Design review of the part built by this model. Coordinates are the model's own, in mm. A direction names the side the tool comes from. Coordinates: 2 decimals unless noted, no trailing zeros. Order: outer loops, then holes, each group sorted by start corner. A loop starts at its lowest first (then second) coordinate and runs counter-clockwise, first axis right, second up. Notation, with made-up numbers: M 42.25,-30 L 51.25,-30 A8 cw 51.25,-18 Z; hole C -19.75,-28.75 d9. An arc over 180 degrees is marked long. Answer in a Markdown table with one row per item.
Autodesk Inventor part; units mm, degrees
ref_plane "Work Plane1" through (0, 21, 0) normal (0, 1, 0) x (1, 0, 0)
ref_plane "YZ Plane" through (0, 0, 0) normal (1, 0, 0) x (0, 1, 0)
ref_plane "XZ Plane" through (0, 0, 0) normal (0, 1, 0) x (-1, 0, 0)
sketch "Sketch1" plane through (0, 0, 0) normal (0, 1, 0) x (-1, 0, 0)
  line L0 (0, 0) -> (20, 0)
  line L1 (20, 0) -> (20, -20)
  line L2 (20, -20) -> (0, -20)
  line L3 (0, -20) -> (0, 0)
  dimension "d0" = 20
  dimension "d1" = 20
extrude "Extrusion1" add sketch "Sketch1" along normal blind 5
sketch "Sketch2" plane through (0, 5, 0) normal (0, 1, 0) x (1, 0, 0)
  line L0 (0, 0) -> (0, 20)
  line L1 (-20, 0) -> (0, 0)
  point P0 (-7.5, 5)
  dimension "d4" = 7.5
  dimension "d55" = 5
hole "Hole1" at (-7.5, 5, -5) direction (0, -1, 0) diameter 6.6 end through all
chamfer "Chamfer1" distance 0.5 angle 45 1 edges at (-7.5, 0, -8.3)
sketch "Sketch3" plane through (0, 5, 0) normal (0, 1, 0) x (1, 0, 0)
  circle A0 centre (-7.5, 5) radius 3.3 construction
  line L0 (0, 20) -> (-20, 20) construction
  line L1 (-20, 20) -> (-20, 0) construction
  line L2 (-20, 0) -> (0, 0) construction
  line L3 (0, 0) -> (0, 20) construction
  line L4 (-20, 20) -> (-20, 0) construction
  line L5 (0, 20) -> (-20, 20) construction
  line L6 (-20, 0) -> (-15, 0)
  line L7 (-15, 0) -> (-15, 20)
  line L8 (-15, 20) -> (-20, 20)
  line L9 (-20, 20) -> (-20, 0)
  line L10 (0, 20) -> (-20, 20)
  line L11 (-20, 20) -> (-20, 10)
  line L12 (-20, 10) -> (0, 10)
  line L13 (0, 10) -> (0, 20)
  point P0 (-15, 10)
  dimension "d56" = 15
  dimension "d57" = 10
extrude "Extrusion2" add sketch "Sketch3" along normal blind 15
sketch "Sketch6" plane through (0, 20, 0) normal (0, 1, 0) x (1, 0, 0)
  line L0 (0, 20) -> (-20, 20) construction
  line L1 (-20, 20) -> (-20, 0) construction
  line L2 (-20, 0) -> (-15, 0) construction
  line L3 (-15, 0) -> (-15, 10) construction
  line L4 (-15, 10) -> (0, 10) construction
  line L5 (0, 10) -> (0, 20) construction
  line L6 (-2.5, 10) -> (-13, 10)
  line L7 (-13, 10) -> (-13, 20)
  line L8 (-13, 20) -> (-2.5, 20)
  line L9 (-2.5, 20) -> (-2.5, 10)
  dimension "d32" = 2.5
  dimension "d33" = 10.5
  dimension "d34" = 2
extrude "Extrusion5" add sketch "Sketch6" along normal blind 3
fillet "Fillet4" radius 2 6 edges at (-13, 23, -15) (-2.5, 23, -15) (0, 2.5, 0) (-20, 10, 0) (0, 10, -20) (-20, 10, -20)
sketch "Sketch7" plane through (0, 5, -10) normal (0, 0, 1) x (1, 0, 0)
  line L0 (-11, 18) -> (-4.5, 18)
  line L1 (0, 0) -> (0, 15)
  point P0 (0, -5)
  point P1 (-7.5, 13)
  dimension "d36" = 5
  dimension "d58" = 7.5
hole "Hole2" at (-7.5, 18, -10) direction (0, 0, -1) diameter 5.5 end through all
fillet "Fillet5" radius 2 2 edges at (-2.5, 20, -15) (-13, 20, -15)
chamfer "Chamfer2" distance 0.2 angle 45 1 edges at (-7.5, 20.75, -10)
ref_plane "Work Plane1" through (0, 21, 0) normal (0, 1, 0) x (1, 0, 0)
sketch "Sketch9" plane through (0, 21, 0) normal (0, 1, 0) x (1, 0, 0)
  line L0 (-15, 10) -> (-15, 0)
  point P0 (0, 0)
hole "Hole4" at (-15, 21, -10) direction (0, -1, 0) diameter 1 depth 16
sketch "Sketch10" plane through (0, 5, -10) normal (1, 0, 0) x (0, 0, -1)
  line L0 (8, 15) -> (8, -5) construction
  line L1 (0, 15) -> (8, 15) construction
  line L2 (0, 0) -> (0, 15) construction
  line L3 (-8, 0) -> (0, 0) construction
  line L4 (-8, -5) -> (-8, 0) construction
  line L5 (-8, -5) -> (8, -5) construction
  line L6 (0, 0) -> (1, 0)
  line L7 (1, 0) -> (1, 4.5)
  line L8 (1, 4.5) -> (0, 4.5)
  line L9 (0, 4.5) -> (0, 0)
  point P0 (-10, -5)
  dimension "d67" = 1
  dimension "d68" = 4.5
extrude "Extrusion6" cut sketch "Sketch10" against normal up to surface (15 mm away)
properties part number "KN-00-02-08" material "X5CrNi18-10"
(1) Add section D-D, the plane z = -16.25. Give the boundary of the cut face in (x, y).
Return value:
| item | result |
|---|---|
| outline | M -20,0 L 0,0 L 0,20 L -0.63,20 A2 cw -2.56,21.5 A2 ccw -4.5,23 L -11,23 A2 ccw -12.94,21.5 A2 cw -14.87,20 L -20,20 Z; hole C -7.5,18 d5.5 |
(2) Add section B-B, the plane y = 18. Give the boundary of the cut face in (x, z), and give its area (3 significant figures).
Return value:
| item | result |
|---|---|
| outline | M -20,-18 A2 ccw -18,-20 L -10.25,-20 L -10.25,-10.2 L -10.45,-10 L -14.5,-10 A0.5 cw long -15,-9.5 L -15,0 L -18,0 A2 ccw -20,-2 Z; M -4.75,-20 L -2,-20 A2 ccw 0,-18 L 0,-10 L -4.55,-10 L -4.75,-10.2 Z |
| area | 192 mm2 |
(3) Add section C-C, the plane y = 3. Give the boundary of the cut face in (x, z).
Return value:
| item | result |
|---|---|
| outline | M -20,-18 A2 ccw -18,-20 L -2,-20 A2 ccw 0,-18 L 0,-2 A2 ccw -2,0 L -18,0 A2 ccw -20,-2 Z; hole C -7.5,-5 d6.6 |
(4) For line 1 along Y through (x, z) = (-7.5, -15); line 2 along X through (y, z) = (18, -15.25); line 3 along X through (y, z) = (15.5, -3.5), list the stretches that pass through material, from the lowest coordinate up. Write a range as from..to.
Return value:
| item | result |
|---|---|
| line 1 | y = 0..15.25, 20.75..23 |
| line 2 | x = -20..-10.25, -4.75..0 |
| line 3 | x = -20..-15 |
(5) Insertion check: pin 1 Ø5.5 at (x, z) = (-16.5, -10) entering from +Y; pin 2 Ø1.5 at (x, y) = (-12, 13.5) entering from +Z; pin 3 Ø3.5 at (x, z) = (-9.5, -7.5) entering from +Y; pin 4 Ø2 at (y, z) = (14.5, -17) entering from +X. Each pin has a flat end and moves straight along its axis. Give the tip position at first contact, or say it passes through.
Return value:
| item | result |
|---|---|
| pin 1 | stops at y = 20.35 |
| pin 2 | stops at z = -10 |
| pin 3 | stops at y = 5 |
| pin 4 | stops at x = 0 |
(6) For faces 1 (the flat face through (-7.4, 14.7, -10)), 2 (the flat face through (-7.4, 9.5, -10.5)), 3 (the flat face through (-17, 20, -10)), 4 (the cylindrical face through (-15.487, 12.412, -10.113)), list the 3-axis set-ups (+Z, -Z, +X, -X, +Y, -Y) from which the entire face can be reached by the end or side of a thin tool; tool diameter is ignored.
Return value:
| item | result |
|---|---|
| face 1 | +Z, +X, +Y |
| face 2 | +Z, +X |
| face 3 | +Z, -Z, -X, +Y |
| face 4 | +Y |
(7) Add section A-A, the plane z = -5. Give the boundary of the cut face in (x, y), and give its area (3 significant figures).
Return value:
| item | result |
|---|---|
| outline | M -20,0 L -11.3,0 L -10.8,0.5 L -10.8,5 L -15,5 L -15,20 L -20,20 Z; M -4.2,0.5 L -3.7,0 L 0,0 L 0,5 L -4.2,5 Z |
| area | 142 mm2 |
(8) Draft analysis for pull direction X (two halves, no side actions). For faces 5 (the flat face through (-7, 7, -11)), 6 (the cylindrical face through (-0.6, 2.54, -0.57)), 7 (the cylindrical face through (-5.827, 20.182, -15.169)), state which applies: pulls with the +X half, pulls with the -X half, needs draft (parallel to the pull), parting line crosses it, or undercut.
Return value:
| item | result |
|---|---|
| face 5 | needs draft |
| face 6 | pulls with the +X half |
| face 7 | undercut |
